CAD build for the part. Positions are in the model's coordinates, mm. A direction names the side the tool comes from. Coordinates: 2 decimals unless noted, no trailing zeros. Write each loop counter-clockwise with the first axis right and the second up, starting at its lowest first coordinate (ties: lowest second). Pieces come first, ordered by that corner, then holes. Notation, with made-up numbers: (39.5, 28) -> (91.5, 28) arc R27 ccw to (91.5, 67) -> close; hole circle Ø1 at (83.5, -19.5). An arc over 180 degrees is marked (long way). Answer as CSV lines item,"result". Start each with the question number.
```python
from build123d import *

# Parameters (mm, degrees)
F1_DEPTH = 38.1
F4_W     = 38.1
F4_H     = 88.9
F4_W_2   = 88.9
F4_H_2   = 38.1
F5_DEPTH = 482.6
F7_DEPTH = 38.1
F8_W     = 88.9
F8_H     = 38.1
F9_DEPTH = 177.8


# Not quite as in the source:
# - a feature names something its author has since deleted; it is built from what else it names


with BuildPart() as f1:
    # F0 (on Front) → F1 (new body)
    with BuildSketch(Plane.XZ):
        Polygon((251.46, 403.1040360442), (251.46, 88.9), (340.36, 88.9), (340.36, 431.8), (340.36, 520.7), (251.46, 520.7), (251.46, 519.1547440658), align=None)
        Polygon((0, 308.15475081), (0, 88.9), (88.9, 88.9), (88.9, 266.7), (251.46, 403.1040360442), (251.46, 519.1547440658), align=None)
        Polygon((0, 88.9), (0, 0), (1257.3, 0), (1257.3, 88.9), (452.2981294842, 88.9), (342.8563937201, 88.9), (340.36, 88.9), (251.46, 88.9), (88.9, 88.9), align=None)
        Polygon((673.1, 431.8), (698.5, 431.8), (698.5, 520.7), (340.36, 520.7), (340.36, 431.8), (589.0582642359, 431.8), align=None)
        Polygon((342.8563937201, 88.9), (452.2981294842, 88.9), (698.5, 431.8), (673.1, 431.8), (589.0582642359, 431.8), align=None)
    extrude(amount=-F1_DEPTH)


with BuildPart() as f3_1:
    # F3: instance of F1
    add(f1.part.mirror(Plane(origin=(466.9868832569, 279.4, 206.694910325), x_dir=(1, 0, 0), z_dir=(0, 1, 0))))


with BuildPart() as f1_1:
    add(f1.part)

    add(f3_1.part)  # F5 merges F3_1
    # F4 (on face) → F5 (join, through all)
    with BuildSketch(Plane(origin=(0, 38.1, 0), x_dir=(-1, 0, 0), z_dir=(0, 1, 0))):
        with Locations((-19.05, 44.45)):
            Rectangle(F4_W, F4_H)
        with Locations((-270.51, 44.45)):
            Rectangle(F4_W, F4_H)
        Polygon((-88.9, 266.7), (-31.7561814989, 334.8013509933), (-60.9424747817, 359.2915589223), (-118.0862932828, 291.1902079291), align=None)
        Polygon((-205.6451731313, 364.6608317162), (-148.5013546302, 432.7621827095), (-177.687647913, 457.2523906386), (-234.8314664142, 389.1510396453), align=None)
        with Locations((-803.91, 44.45)):
            Rectangle(F4_W, F4_H)
        Polygon((-251.46, 482.6), (-251.46, 519.1547440658), (-251.46, 520.7), (-340.36, 520.7), (-340.36, 482.6), align=None)
        with Locations((-1223.01, 44.45)):
            Rectangle(F4_W, F4_H)
        with Locations((-654.05, 501.65)):
            Rectangle(F4_W_2, F4_H_2)
    extrude(amount=F5_DEPTH)

    # F6 (on face) → F7 (join)
    with BuildSketch(Plane(origin=(0, 558.8, 0), x_dir=(-1, 0, 0), z_dir=(0, 1, 0))):
        Polygon((-646.6455672201, 359.5792448815), (-698.5, 431.8), (-1190.2829408646, 88.9), (-1034.85039393, 88.9), align=None)
    extrude(amount=-F7_DEPTH)

    # F8 (on face) → F9 (join)
    with BuildSketch(Plane(origin=(0, 558.8, 0), x_dir=(-1, 0, 0), z_dir=(0, 1, 0))):
        with Locations((-789.2684733582, 318.4677249113)):
            Rectangle(F8_W, F8_H)
    extrude(amount=F9_DEPTH)


solid = f1_1.part
```
1. Tool access for faces 5 (the face through (19, 276, 88.9)), 6 (the face through (89.11, 276.02, 325.72)), 7 (the face through (177.5, 276, 398.2)), 8 (the face through (340.36, 276, 502)): list every direction of +Z, -Z, +X, -X, +Y, -Y with a clear straight run to the whole face (end or side of a thin tool).
2. Flat gauge pins, fed straight in: P1, Ø11.5, axis at y = 542, z = 260, coming from the +X side; P2, Ø8, axis at x = 231.5, y = 469, coming from the +Z side; P3, Ø8, axis at x = 817.5, y = 628, coming from the -Z side. Where does each tip first touch, or does it go through?
3. Mould opens along X. For faces 1 (the face through (790, 736.6, 319)), 2 (the face through (171, 540, 88.9)), 3 (the face through (1242.06, 276, 44)), 4 (the face through (467.68, 540.02, 262.75)) say: pulls with the +X half, pulls with the -X half, needs draft (parallel to the pull), parting line crosses it, or undercut.
4. Cut at A-A (y = 85). Count the separate pieces of the cut face and the enclosed holes in it, then the cut area to 3 significant figures.
5. Cut at C-C (x = 437). Give the cut face in (y, z).
6. Cut at D-D (x = 1075). Give the cut face in (y, z), then the cut area to 3 significant figures.
7. Cut at B-B (z = 138). Give the cut face in (x, y).
8. Wall check: line 1 (Y direction, x = 290.5, z = 213.5); line 2 (X direction, y = 527, z = 270); line 3 (Z direction, x = 412, y = 532). Give the ranges that are in metal, low to high.
Geometry check:
1,face 5,"+X, -X"
1,face 6,"+Z, +X"
1,face 7,"-Z, -X"
1,face 8,"+Z, -Z"
2,P1,"x = 953.14"
2,P2,"z = 397.89"
2,P3,"z = 299.42"
3,face 1,"needs draft"
3,face 2,"undercut"
3,face 3,"pulls with the +X half"
3,face 4,"undercut"
4,separate pieces,"8"
4,enclosed holes,"0"
4,area,"27,100 mm²"
5,outline,"(0, 0) -> (38.1, 0) -> (38.1, 220.02) -> (0, 220.02) -> close; (0, 431.8) -> (38.1, 431.8) -> (38.1, 520.7) -> (0, 520.7) -> close; (520.7, 0) -> (558.8, 0) -> (558.8, 220.02) -> (520.7, 220.02) -> close; (520.7, 431.8) -> (558.8, 431.8) -> (558.8, 520.7) -> (520.7, 520.7) -> close"
6,outline,"(0, 0) -> (38.1, 0) -> (38.1, 88.9) -> (0, 88.9) -> close; (520.7, 0) -> (558.8, 0) -> (558.8, 169.28) -> (520.7, 169.28) -> close"
6,area,"9,840 mm²"
7,outline,"(0, 0) -> (88.9, 0) -> (88.9, 38.1) -> (0, 38.1) -> close; (0, 520.7) -> (88.9, 520.7) -> (88.9, 558.8) -> (0, 558.8) -> close; (251.46, 0) -> (340.36, 0) -> (340.36, 38.1) -> (251.46, 38.1) -> close; (251.46, 520.7) -> (340.36, 520.7) -> (340.36, 558.8) -> (251.46, 558.8) -> close; (378.11, 0) -> (487.55, 0) -> (487.55, 38.1) -> (378.11, 38.1) -> close; (378.11, 520.7) -> (487.55, 520.7) -> (487.55, 558.8) -> (378.11, 558.8) -> close; (964.43, 520.7) -> (1119.86, 520.7) -> (1119.86, 558.8) -> (964.43, 558.8) -> close"
8,line 1,"0 to 38.1, 520.7 to 558.8"
8,line 2,"0 to 92.83, 251.46 to 340.36, 472.89 to 582.33, 775.12 to 930.55"
8,line 3,"0 to 185.2, 431.8 to 520.7"
